Here's how the part is built. I have some questions about the finished solid (model axes, mm). Round coordinates to 2 decimals unless told otherwise and drop trailing zeros. Write each loop counter-clockwise with the first axis right and the second up, starting at its lowest first coordinate (ties: lowest second). Pieces come first, ordered by that corner, then holes. Notation, with made-up numbers: (15, 13) - (57, 13) arc R31 cw to (57, 44) - close; hole circle Ø8 at (-14, 47). An arc over 180 degrees is marked (long way). Return JSON: item names as keys, results as strings. Group by question number.
```python
from build123d import *

# Parameters (mm, degrees)
BOX057_W          = 10
BOX057_H          = 2.5
BOX057_DEPTH      = 10
CYLINDER064_R     = 10.3
CYLINDER064_DEPTH = 10


with BuildPart() as cube056:
    # Box057 → Box057 (new body)
    with BuildSketch(Plane(origin=(85.7, 163.75, -5), x_dir=(1, 0, 0), z_dir=(0, 0, 1))):
        with Locations((5, 1.25)):
            Rectangle(BOX057_W, BOX057_H)
    extrude(amount=BOX057_DEPTH)


with BuildPart() as obj1:
    # Cylinder064 → Cylinder064 (new body)
    with BuildSketch(Plane(origin=(85, 165, -5), x_dir=(1, 0, 0), z_dir=(0, 0, 1))):
        Circle(CYLINDER064_R)
    extrude(amount=CYLINDER064_DEPTH)

    # Fusion009: union Cube056
    add(cube056.part)


with BuildPart() as obj1_1:
    # Fusion009 placement: moved
    add(obj1.part.moved(Location((6.5, 15, 0))))


solid = obj1_1.part
```
1) Imagine slicing it at B-B (y = 172.5). Please give me the cut outline in (x, z), plus the area to 3 significant figures.
2) Will these pins go through, and if not, where does the flat tip stop? pin 1 Ø3 at (y, z) = (187, 4) entering from -X; pin 2 Ø5 at (y, z) = (186, 1.5) entering from +X; pin 3 Ø2 at (x, z) = (94.5, 0.5) entering from -Y.
3) Imagine slicing it at A-A (z = 0.75). Please give me the cut outline in (x, y).
4) I need wall thicknesses on line 1 along Y through (x, z) = (91.75, -4.25); line 2 along X through (y, z) = (183, -1); line 3 along X through (y, z) = (179.25, 2.5). Which ranges of each line are inside material? Lowest first, please.
Results found:
{
 "1": {"outline": "(84.44, -5) - (98.56, -5) - (98.56, 5) - (84.44, 5) - close", "area": "141 mm²"},
 "2": {"pin 1": "stops at x = 82.79", "pin 2": "stops at x = 101.19", "pin 3": "stops at y = 169.9"},
 "3": {"outline": "(101.72, 178.75) - (102.2, 178.75) - (102.2, 181.25) - (101.72, 181.25) arc R10.3 ccw (long way) to start"},
 "4": {"line 1": "y = 169.7 to 190.3", "line 2": "x = 81.65 to 101.35", "line 3": "x = 81.23 to 102.2"}
}
